Check sheet for the drawn part. Datum: minimum x, y, z corner. Units: mm. A direction names the side the tool comes from. Round coordinates to 2 decimals unless told otherwise and drop trailing zeros. Order: outer loops, then holes, each group sorted by start corner. A loop starts at its lowest first (then second) coordinate and runs counter-clockwise, first axis right, second up. Notation, with made-up numbers: M 89,2.5 L 135,2.5 A14 ccw 135,26.5 Z; hole C 38.25,75 d1. An arc over 180 degrees is marked long. Write item = value, one per line. Start each with the question number.
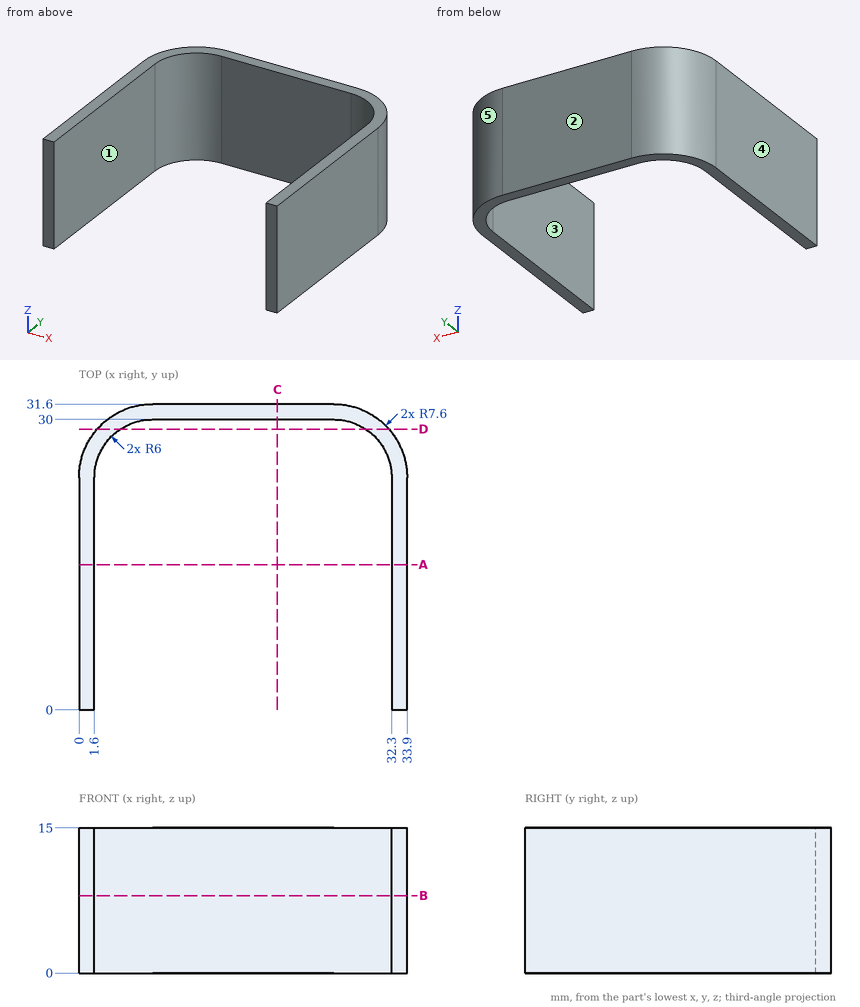
1) Access from +Z, -Z, +X, -X, +Y, -Y to the whole of each face (thin tool, end or side, straight path). Record for the marked faces 1 and 2.
2) Release check for a two-part mould opening along X. For the marked faces 3, 4 and 5 record: pulls with the +X half, pulls with the -X half, needs draft (parallel to the pull), parting line crosses it, or undercut.
3) Gauge pin test, flat ends, axial feed: P1, Ø5, axis at x = 7.5, z = 9.5, coming from the -Y side; P2, Ø8, axis at x = 26, z = 4.5, coming from the -Y side; P3, Ø1, axis at x = 27, z = 4, coming from the +Y side; P4, Ø10, axis at x = 15, y = 26.5, coming from the +Z side. Record the tip position at first contact, or that the pin passes through.
4) Cross-section at D-D, the plane y = 29. Enter the section's corners in (x, z), then the cut area to 3 significant figures.
5) Scan lines: probe 1 along X at (y, z) = (13.5, 3.25); probe 2 along Y at (x, z) = (23.5, 7.25); probe 3 along X at (y, z) = (28.5, 10.75). Record each from-to range of solid material in increasing order.
6) Cross-section at C-C, the plane x = 20.5. Enter the section's corners in (y, z), then the cut area to 3 significant figures.
7) Cross-section at A-A, the plane y = 15. Enter the section's corners in (x, z), then the cut area to 3 significant figures.
8) Cross-section at B-B, the plane z = 8. Enter the section's corners in (x, y), then the cut area to 3 significant figures.
Geometry results:
q1.face_1 = +Z, -Z, -Y
q1.face_2 = +Z, -Z, +X, -X, +Y
q2.face_3 = undercut
q2.face_4 = pulls with the -X half
q2.face_5 = pulls with the +X half
q3.P1 = 29.41
q3.P2 = 28.72
q3.P3 = 31.6
q3.P4 = 15
q4.outline = M 1.88,0 L 4.28,0 L 4.28,15 L 1.88,15 Z; M 29.62,0 L 32.02,0 L 32.02,15 L 29.62,15 Z
q4.area = 72.2 mm^2
q5.probe_1 = 0 to 1.6, 32.3 to 33.9
q5.probe_2 = 30 to 31.6
q5.probe_3 = 1.48 to 3.63, 30.27 to 32.42
q6.outline = M 30,0 L 31.6,0 L 31.6,15 L 30,15 Z
q6.area = 24.0 mm^2
q7.outline = M 0,0 L 1.6,0 L 1.6,15 L 0,15 Z; M 32.3,0 L 33.9,0 L 33.9,15 L 32.3,15 Z
q7.area = 48.0 mm^2
q8.outline = M 0,0 L 1.6,0 L 1.6,24 A6 cw 7.6,30 L 26.3,30 A6 cw 32.3,24 L 32.3,0 L 33.9,0 L 33.9,24 A7.6 ccw 26.3,31.6 L 7.6,31.6 A7.6 ccw 0,24 Z
q8.area = 141 mm^2
